from build123d import *

# Parameters (mm, degrees)
PAD_DEPTH    = 0.375
SKETCH002_R  = 1.5
PAD001_DEPTH = 0.5
SKETCH003_R  = 0.6
PAD002_DEPTH = 0.3
SKETCH004_R  = 0.15
PAD003_DEPTH = 0.5
SKETCH005_R  = 0.6
PAD004_DEPTH = 0.3


with BuildPart() as part:
    # Sketch → Pad (new body, symmetric)
    with BuildSketch(Plane.XY):
        with BuildLine():
            Line((-0.25, 0), (0, 0))
            Line((0, 0), (0.25, 0))
            ThreePointArc((0.25, 0), (8.963573, -21.036427), (30, -29.75))
            Line((30, -29.75), (30, -30))
            Line((30, -30), (30, -30.25))
            ThreePointArc((-0.25, 0), (8.61002, -21.38998), (30, -30.25))
        make_face()
    extrude(amount=PAD_DEPTH, both=True)

    # Sketch002 → Pad001 (join)
    with BuildSketch(Plane.XZ):
        Circle(SKETCH002_R)
    extrude(amount=PAD001_DEPTH)

    # Sketch003 (on DatumPlane) → Pad002 (join)
    with BuildSketch(Plane(origin=(30, -30, 0), x_dir=(0, 1, 0), z_dir=(1, 0, 0))):
        Circle(SKETCH003_R)
    extrude(amount=PAD002_DEPTH)

    # Sketch004 (on DatumPlane) → Pad003 (join)
    with BuildSketch(Plane(origin=(30.3, -30, 0), x_dir=(0, 1, 0), z_dir=(1, 0, 0))):
        Circle(SKETCH004_R)
    extrude(amount=PAD003_DEPTH)

    # Sketch005 (on DatumPlane) → Pad004 (join)
    with BuildSketch(Plane(origin=(30.8, -30, 0), x_dir=(0, 1, 0), z_dir=(1, 0, 0))):
        Circle(SKETCH005_R)
    extrude(amount=PAD004_DEPTH)


solid = part.part
Geometry: final body of the model. Coordinates: model frame, mm. A direction names the side the tool comes from. Give positions to 0.01 mm unless a question says otherwise; leave off trailing zeros. Write each loop counter-clockwise with the first axis right and the second up, starting at its lowest first coordinate (ties: lowest second). Pieces come first, ordered by that corner, then holes. Notation, with made-up numbers: (0.25, 23) -> (59.25, 23) arc R13 cw to (59.25, 39) -> close; hole circle Ø5 at (87, 5). An arc over 180 degrees is marked (long way). Answer in a Markdown table with one row per item.
(1) Draft query along X for faces 1 (the flat face through (13.8, -25.2, -0.375)), 2 (the flat face through (30.3, -29.7, 0)), 3 (the cylindrical face through (8.55, -21.33, 0.01)). Return one class per face: +X half, -X half, draft (parallel to the pull), parting line (faces both ways), or undercut.
Answers below:
| item | result |
|---|---|
| face 1 | draft |
| face 2 | undercut |
| face 3 | -X half |
(2) Set-up query: faces 4 (the flat face through (31.1, -30, 0)), 5 (the flat face through (13.8, -25.2, 0.375)), 6 (the flat face through (30.8, -29.7, 0)). Return all of +Z, -Z, +X, -X, +Y, -Y with unobstructed straight access to the full face (end or side cutting, diameter ignored); none if empty.
Answers below:
| item | result |
|---|---|
| face 4 | +Z, -Z, +X, +Y, -Y |
| face 5 | +Z, -X, -Y |
| face 6 | none |
(3) Pin query (flat end, axial travel): pin 1 (15 mm diameter, centred on x = 15, y = -14, fed in from -Z); pin 2 (4 mm diameter, centred on x = 13.5, y = -24, fed in from +Z) (3 decimals); pin 3 (2 mm diameter, centred on x = 15, y = -26, fed in from -Z) (3 decimals). Return the tip coordinate at first contact, or that it passes through.
Answers below:
| item | result |
|---|---|
| pin 1 | through |
| pin 2 | z = 0.375 |
| pin 3 | z = -0.375 |
(4) Section query B-B on y = -28. Return loops of the section in (x, z) (3 decimals).
Answers below:
| item | result |
|---|---|
| outline | (18.552, -0.375) -> (19.947, -0.375) -> (19.947, 0.375) -> (18.552, 0.375) -> close |
(5) Section query A-A on x = 1. Return loops of the section in (y, z) (3 decimals).
Answers below:
| item | result |
|---|---|
| outline | (-8.606, -0.375) -> (-6.638, -0.375) -> (-6.638, 0.375) -> (-8.606, 0.375) -> close; (-0.5, -1.118) -> (0, -1.118) -> (0, 1.118) -> (-0.5, 1.118) -> close |
(6) Section query C-C on x = 8. Return loops of the section in (y, z) (3 decimals), then the cut area to 3 significant figures.
Answers below:
| item | result |
|---|---|
| outline | (-20.762, -0.375) -> (-20.027, -0.375) -> (-20.027, 0.375) -> (-20.762, 0.375) -> close |
| area | 0.552 mm^2 |
(7) Ray query, line 1 along Y through (x, z) = (8, 0.3); line 2 along Y through (x, z) = (20, -0.25). Return the intervals inside material, ascending. Write a range as [from, to].
Answers below:
| item | result |
|---|---|
| line 1 | [-20.76, -20.03] |
| line 2 | [-28.55, -28.02] |
